The listing builds one solid part. Answer for the finished solid, in the listing's coordinates (mm). Round coordinates to 2 decimals unless told otherwise and drop trailing zeros. Write each loop counter-clockwise with the first axis right and the second up, starting at its lowest first coordinate (ties: lowest second). Pieces come first, ordered by that corner, then holes.
Item 1: Find section D-D on x = -6. Give the vertices of the cut face in (y, z), then the cut area to 3 significant figures.
Item 2: Find the intervals of material crossed by probe 1 along X at (y, z) = (20.25, 1.6); probe 2 along X at (y, z) = (5, 1.6); probe 3 along Y at (x, z) = (-7, 1), in increasing order.
Item 3: Each of these flat-tipped pins is pushed along its axis until it touches: pin 1 (1.6 mm diameter, centred on x = 7.5, y = 1.5, fed in from +Z); pin 2 (1.5 mm diameter, centred on x = -13.5, y = 7.5, fed in from -Z); pin 3 (1 mm diameter, centred on x = -13, z = 1, fed in from +Y). Where does it stop, or does it pass through?
Item 4: Find section B-B on z = 1. Give the vertices of the cut face in (x, y), then the cut area to 3 significant figures.
Item 5: Find section A-A on y = 14.75. Give the vertices of the cut face in (x, z), then the cut area to 3 significant figures.
Item 6: Find section C-C on y = 4. Give the vertices of the cut face in (x, z), then the cut area to 3 significant figures.
```python
from build123d import *

# Parameters (mm, degrees)
SKETCH2_W             = 4
SKETCH2_H             = 28
BOSS_EXTRUDE1_DEPTH   = 2
BOSS_EXTRUDE1_2_DEPTH = 2
SKETCH3_W             = 16
SKETCH3_H             = 2
BOSS_EXTRUDE2_DEPTH   = 0.4
SKETCH7_W             = 2
SKETCH7_H             = 14
BOSS_EXTRUDE3_DEPTH   = 18
SKETCH6_R             = 0.36
CUT_EXTRUDE1_DEPTH    = 35


with BuildPart() as part:
    # Sketch2 → Boss-Extrude1 (new body)
    with BuildSketch(Plane.XY):
        with Locations((2, 14)):
            Rectangle(SKETCH2_W, SKETCH2_H)
    extrude(amount=BOSS_EXTRUDE1_DEPTH)



with BuildPart() as body_2:
    # Sketch2 → Boss-Extrude1 2 (new body)
    with BuildSketch(Plane.XY):
        with Locations((14, 14)):
            Rectangle(SKETCH2_W, SKETCH2_H)
    extrude(amount=BOSS_EXTRUDE1_2_DEPTH)


with BuildPart() as part_1:
    add(part.part)

    add(body_2.part)  # Boss-Extrude2 merges body 2
    # Sketch3 → Boss-Extrude2 (add)
    with BuildSketch(Plane(origin=(0, 0, 0), x_dir=(-1, 0, 0), z_dir=(0, 0, -1))):
        with Locations((-8, 1)):
            Rectangle(SKETCH3_W, SKETCH3_H)
    extrude(amount=-BOSS_EXTRUDE2_DEPTH)

    # Sketch7 → Boss-Extrude3 (add)
    with BuildSketch(Plane.ZY):
        with Locations((1, 7)):
            Rectangle(SKETCH7_W, SKETCH7_H)
    extrude(amount=BOSS_EXTRUDE3_DEPTH)

    # Sketch6 → Cut-Extrude1 (cut, through all)
    with BuildSketch(Plane(origin=(16, 0, 0), x_dir=(0, 0, -1), z_dir=(1, 0, 0))):
        with Locations((-1, 4)):
            Circle(SKETCH6_R)
    extrude(amount=-CUT_EXTRUDE1_DEPTH, mode=Mode.SUBTRACT)


solid = part_1.part
```
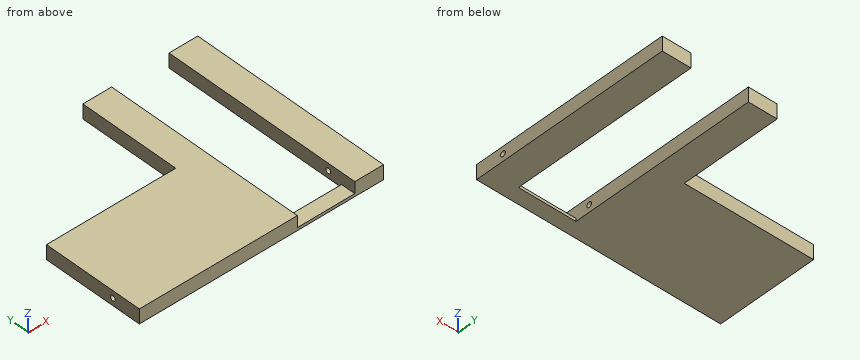
Check values:
1. outline: (0, 0) - (14, 0) - (14, 2) - (0, 2) - close; hole circle Ø0.72 at (4, 1)
1. area: 27.6 mm2
2. probe 1: x = 0 to 4, 12 to 16
2. probe 2: x = -18 to 4, 12 to 16
2. probe 3: y = 0 to 3.64, 4.36 to 14
3. pin 1: stops at z = 0.4
3. pin 2: stops at z = 0
3. pin 3: stops at y = 14
4. outline: (-18, 0) - (4, 0) - (4, 3.64) - (-18, 3.64) - close; (-18, 4.36) - (4, 4.36) - (4, 28) - (0, 28) - (0, 14) - (-18, 14) - close; (12, 0) - (16, 0) - (16, 3.64) - (12, 3.64) - close; (12, 4.36) - (16, 4.36) - (16, 28) - (12, 28) - close
4. area: 457 mm2
5. outline: (0, 0) - (4, 0) - (4, 2) - (0, 2) - close; (12, 0) - (16, 0) - (16, 2) - (12, 2) - close
5. area: 16.0 mm2
6. outline: (-18, 0) - (4, 0) - (4, 0.64) - (-18, 0.64) - close; (-18, 1.36) - (4, 1.36) - (4, 2) - (-18, 2) - close; (12, 0) - (16, 0) - (16, 0.64) - (12, 0.64) - close; (12, 1.36) - (16, 1.36) - (16, 2) - (12, 2) - close
6. area: 33.3 mm2
